Job drawing, mm, ordinate dimensions from the low corner. One solid piece. Round coordinates to 2 decimals unless told otherwise and drop trailing zeros. Write each loop counter-clockwise with the first axis right and the second up, starting at its lowest first coordinate (ties: lowest second). Pieces come first, ordered by that corner, then holes. Notation, with made-up numbers: (-37.5, 10.5) - (20.5, 10.5) arc R26 ccw to (20.5, 30.5) - close; hole circle Ø4 at (1, -14). An arc over 180 degrees is marked (long way). Write each question's results on one line, items separated by ' | '.
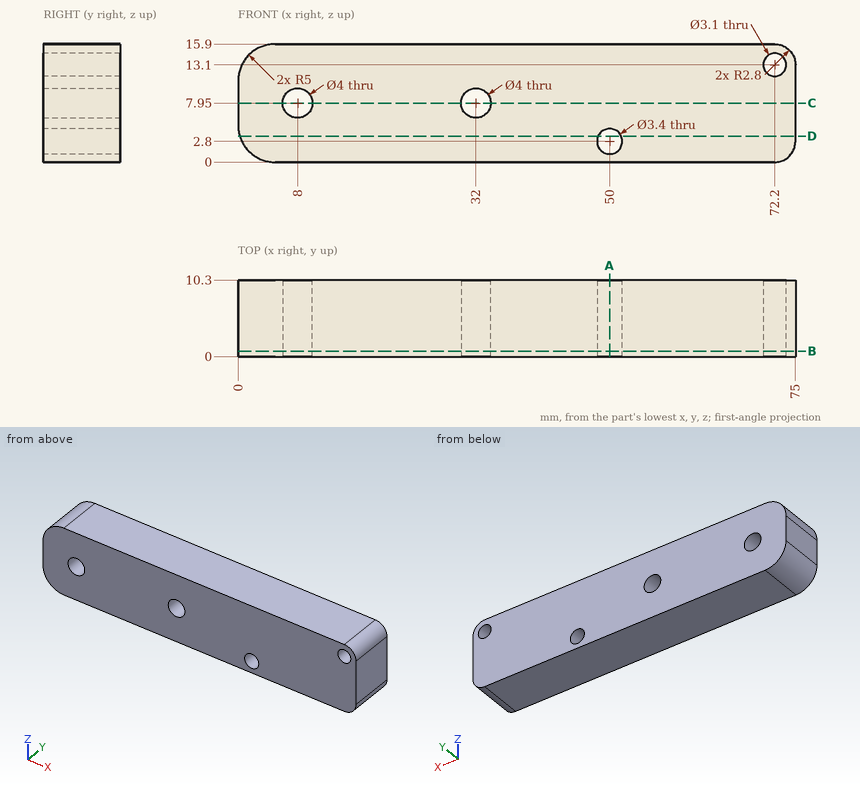
(1) Slice it at B-B, the plane y = 0.75. Write the cut outline in (x, z).
Worked answers:
outline: (0, 5) arc R5 ccw to (5, 0) - (72.2, 0) arc R2.8 ccw to (75, 2.8) - (75, 13.1) arc R2.8 ccw to (72.2, 15.9) - (5, 15.9) arc R5 ccw to (0, 10.9) - close; hole circle Ø4 at (8, 7.95); hole circle Ø4 at (32, 7.95); hole circle Ø3.4 at (50, 2.8); hole circle Ø3.1 at (72.2, 13.1)
(2) Flat gauge pins, fed straight in: pin 1 Ø3 at (x, z) = (50, 2.8) entering from +Y; pin 2 Ø1 at (y, z) = (6, 2) entering from +X. Where does each tip first touch, or does it go through?
Worked answers:
pin 1: passes through | pin 2: stops at x = 74.98
(3) Slice it at A-A, the plane x = 50. Write the cut outline in (y, z).
Worked answers:
outline: (0, 0) - (10.3, 0) - (10.3, 1.1) - (0, 1.1) - close; (0, 4.5) - (10.3, 4.5) - (10.3, 15.9) - (0, 15.9) - close
(4) Slice it at D-D, the plane z = 3.5. Write the cut outline in (x, y), and give its area (3 significant figures).
Worked answers:
outline: (0.23, 0) - (48.45, 0) - (48.45, 10.3) - (0.23, 10.3) - close; (51.55, 0) - (75, 0) - (75, 10.3) - (51.55, 10.3) - close | area: 738 mm2
(5) Slice it at C-C, the plane z = 7.95. Write the cut outline in (x, y).
Worked answers:
outline: (0, 0) - (6, 0) - (6, 10.3) - (0, 10.3) - close; (10, 0) - (30, 0) - (30, 10.3) - (10, 10.3) - close; (34, 0) - (75, 0) - (75, 10.3) - (34, 10.3) - close
(6) Drill centre lines: probe 1 along Z at (x, y) = (50, 5.25); probe 2 along X at (y, z) = (9, 7.25); probe 3 along X at (y, z) = (3, 14.25). Where is each one in solid material? Low to high. Write a range as [from, to].
Worked answers:
probe 1: z = [0, 1.1], [4.5, 15.9] | probe 2: x = [0, 6.13], [9.87, 30.13], [33.87, 75] | probe 3: x = [1.29, 71.16], [73.24, 74.75]
